Can you work these out from the model? Positions are in its coordinate system, mm. Face numbers are marked on the shaded views. A direction names the side the tool comes from. Give positions to 0.01 mm unless a question says otherwise; leave off trailing zeros. Loops run counter-clockwise (first coordinate to the right, second up) from the corner with the lowest first, then second, coordinate; pieces in that order, holes last. Notation, with made-up numbers: (-35.75, -10.5) -> (-27.75, -10.5) arc R25 cw to (-27.75, 20.5) -> close; hole circle Ø1 at (16.25, 67). An arc over 180 degrees is marked (long way). Return JSON: item names as keys, results as strings. Group by question number.
Q1. Will these pins go through, and if not, where does the flat tip stop? pin 1 (0.6 mm diameter, centred on x = 0.5, y = 4.5, fed in from +Z); pin 2 (6 mm diameter, centred on x = -1.5, y = 2.5, fed in from -Z); pin 3 (1.5 mm diameter, centred on y = -2.5, z = 11, fed in from -X); pin 4 (1.5 mm diameter, centred on y = 4, z = 11, fed in from +X).
Q2. Which directions (+Z, -Z, +X, -X, +Y, -Y) give clear straight access to the entire face, cutting with the end or side of a thin tool? Please do the marked faces 4, 5 and 6.
Q3. Suppose I cut it at B-B, the plane z = 10.25. Please give me the cut outline in (x, y), and give its area (3 significant figures).
Q4. Suppose I cut it at D-D, the plane z = 1. Please give me the cut outline in (x, y).
Q5. I need wall thicknesses on line 1 along Y through (x, z) = (-4.5, 12.75); line 2 along X through (y, z) = (0, 12.5); line 3 along Y through (x, z) = (0, 6.5). Which ranges of each line are inside material? Lowest first, please. Write a range as [from, to].
Q6. Suppose I cut it at C-C, the plane z = 13.25. Count the separate pieces of the cut face and the enclosed holes in it, and give its area (3 significant figures).
Q7. Thinking about a two-plate mould opening in X: for the marked faces 1, 2 and 3, which applies, pulls with the +X half, pulls with the -X half, needs draft (parallel to the pull), parting line crosses it, or undercut?
Q8. Suppose I cut it at A-A, the plane y = 0. Please give me the cut outline in (x, z).
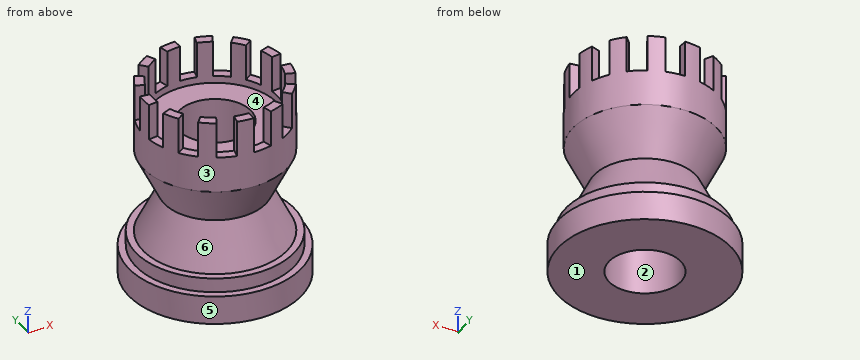
```python
from build123d import *

# Parameters (mm, degrees)
SKETCH_1_R          = 6
EXTRUDE_1_DEPTH     = 2
SKETCH_2_R          = 5.5
EXTRUDE_2_DEPTH     = 1
SKETCH_3_R          = 5
EXTRUDE_3_DEPTH     = 3
EXTRUDE_3_TAPER     = 26
SKETCH_4_R          = 3.536802234
EXTRUDE_4_DEPTH     = 3
EXTRUDE_4_DRAFT     = -26
SKETCH_5_R          = 5
EXTRUDE_5_DEPTH     = 5
SKETCH_6_R          = 4.35308232
CUT_EXTRUDE_1_DEPTH = 3
CUT_EXTRUDE_2_DEPTH = 2.5
SKETCH_8_R          = 2.5
CUT_EXTRUDE_3_DEPTH = 14.892443989


with BuildPart() as part:
    # 스케치1 → 보스-돌출1 (new body)
    with BuildSketch(Plane.XY):
        Circle(SKETCH_1_R)
    extrude(amount=EXTRUDE_1_DEPTH)

    # 스케치2 → 보스-돌출2 (add)
    with BuildSketch(Plane.XY.offset(2)):
        Circle(SKETCH_2_R)
    extrude(amount=EXTRUDE_2_DEPTH)

    # 스케치3 → 보스-돌출3 (add)
    with BuildSketch(Plane.XY.offset(3)):
        Circle(SKETCH_3_R)
    extrude(amount=EXTRUDE_3_DEPTH, taper=EXTRUDE_3_TAPER)


with BuildPart() as extrude_4_tool:
    # 스케치4 → 보스-돌출4 (with draft: the straight prism first)
    with BuildSketch(Plane.XY.offset(6)):
        Circle(SKETCH_4_R)
    extrude(amount=EXTRUDE_4_DEPTH)
    # 보스-돌출4: the draft: its side faces are tilted about the plane it starts from
    extrude_4_sides = [extrude_4_tool.faces().sort_by_distance(p)[0] for p in [
        (-3.536802234, 0, 7.5),
    ]]
    draft(extrude_4_sides, Plane.XY.offset(6), EXTRUDE_4_DRAFT)


with BuildPart() as part_1:
    add(part.part)

    # 보스-돌출4: add extrude_4_tool
    add(extrude_4_tool.part)

    # 스케치5 → 보스-돌출5 (add)
    with BuildSketch(Plane.XY.offset(9)):
        Circle(SKETCH_5_R)
    extrude(amount=EXTRUDE_5_DEPTH)

    # 스케치6 → 컷-돌출1 (cut)
    with BuildSketch(Plane.XY.offset(14)):
        Circle(SKETCH_6_R)
    extrude(amount=-CUT_EXTRUDE_1_DEPTH, mode=Mode.SUBTRACT)

    # 스케치7 → 컷-돌출2 (cut)
    with BuildSketch(Plane.XY.offset(14)):
        with BuildLine():
            Line((0, 4.35308232), (0, 5))
            ThreePointArc((0, 5), (0.642664488, 4.958526228), (1.274667489, 4.834792942))
            Line((1.274667489, 4.834792942), (1.109746502, 4.209250336))
            ThreePointArc((1.109746502, 4.209250336), (0.559514284, 4.316974572), (0, 4.35308232))
        make_face()
        with BuildLine():
            Line((2.022978224, 3.854462971), (2.32361586, 4.427280128))
            ThreePointArc((2.32361586, 4.427280128), (2.873393181, 4.091895847), (3.375502321, 3.688629025))
            Line((3.375502321, 3.688629025), (2.938767895, 3.211381159))
            ThreePointArc((2.938767895, 3.211381159), (2.501623411, 3.562471894), (2.022978224, 3.854462971))
        make_face()
        with BuildLine():
            Line((3.582516517, 2.472832606), (4.114919329, 2.840323734))
            ThreePointArc((4.114919329, 2.840323734), (4.445862124, 2.287861441), (4.70305025, 1.697444651))
            Line((4.70305025, 1.697444651), (4.094552979, 1.47782326))
            ThreePointArc((4.094552979, 1.47782326), (3.870640762, 1.991849838), (3.582516517, 2.472832606))
        make_face()
        with BuildLine():
            Line((4.321343449, 0.524706092), (4.96354437, 0.602683401))
            ThreePointArc((4.96354437, 0.602683401), (4.999837633, -0.04029445), (4.953186046, -0.682603837))
            Line((4.953186046, -0.682603837), (4.312325321, -0.594286139))
            ThreePointArc((4.312325321, -0.594286139), (4.352940961, -0.035081012), (4.321343449, 0.524706092))
        make_face()
        with BuildLine():
            Line((4.070202675, -1.543624265), (4.675081213, -1.773024435))
            ThreePointArc((4.675081213, -1.773024435), (4.408410595, -2.359219368), (4.06860661, -2.906276011))
            Line((4.06860661, -2.906276011), (3.542195901, -2.530251744))
            ThreePointArc((3.542195901, -2.530251744), (3.838034844, -2.053975224), (4.070202675, -1.543624265))
        make_face()
        with BuildLine():
            Line((2.88662752, -3.258328904), (3.315613291, -3.742553741))
            ThreePointArc((3.315613291, -3.742553741), (2.807069816, -4.137675561), (2.251958432, -4.464155376))
            Line((2.251958432, -4.464155376), (1.960592088, -3.886567168))
            ThreePointArc((1.960592088, -3.886567168), (2.443881198, -3.602328466), (2.88662752, -3.258328904))
        make_face()
        with BuildLine():
            Line((1.041760787, -4.22658966), (1.196578321, -4.854709087))
            ThreePointArc((1.196578321, -4.854709087), (0.562663172, -4.968240147), (-0.080586283, -4.999350543))
            Line((-0.080586283, -4.999350543), (-0.070159745, -4.352516892))
            ThreePointArc((-0.070159745, -4.352516892), (0.489863821, -4.325431669), (1.041760787, -4.22658966))
        make_face()
        with BuildLine():
            Line((-1.041760787, -4.22658966), (-1.196578321, -4.854709087))
            ThreePointArc((-1.196578321, -4.854709087), (-1.810642825, -4.660640789), (-2.394669653, -4.389254749))
            Line((-2.394669653, -4.389254749), (-2.084838826, -3.82135745))
            ThreePointArc((-2.084838826, -3.82135745), (-1.576375454, -4.057630604), (-1.041760787, -4.22658966))
        make_face()
        with BuildLine():
            Line((-2.88662752, -3.258328904), (-3.315613291, -3.742553741))
            ThreePointArc((-3.315613291, -3.742553741), (-3.76915237, -3.285344793), (-4.160163063, -2.773633589))
            Line((-4.160163063, -2.773633589), (-3.621906456, -2.414771068))
            ThreePointArc((-3.621906456, -2.414771068), (-3.281486109, -2.860275267), (-2.88662752, -3.258328904))
        make_face()
        with BuildLine():
            Line((-4.070202675, -1.543624265), (-4.675081213, -1.773024435))
            ThreePointArc((-4.675081213, -1.773024435), (-4.864194531, -1.157415898), (-4.972613252, -0.522606399))
            Line((-4.972613252, -0.522606399), (-4.329238966, -0.454989735))
            ThreePointArc((-4.329238966, -0.454989735), (-4.234847844, -1.007665336), (-4.070202675, -1.543624265))
        make_face()
        with BuildLine():
            Line((-4.321343449, 0.524706092), (-4.96354437, 0.602683401))
            ThreePointArc((-4.96354437, 0.602683401), (-4.844908345, 1.235663031), (-4.645897671, 1.848143618))
            Line((-4.645897671, 1.848143618), (-4.044795002, 1.609024262))
            ThreePointArc((-4.044795002, 1.609024262), (-4.218056972, 1.075788579), (-4.321343449, 0.524706092))
        make_face()
        with BuildLine():
            Line((-3.582516517, 2.472832606), (-4.114919329, 2.840323734))
            ThreePointArc((-4.114919329, 2.840323734), (-3.715712045, 3.345666451), (-3.254862922, 3.795506206))
            Line((-3.254862922, 3.795506206), (-2.833737248, 3.304430192))
            ThreePointArc((-2.833737248, 3.304430192), (-3.234960082, 2.912792296), (-3.582516517, 2.472832606))
        make_face()
        with BuildLine():
            Line((-2.022978224, 3.854462971), (-2.32361586, 4.427280128))
            ThreePointArc((-2.32361586, 4.427280128), (-1.735290894, 4.689218007), (-1.118178304, 4.873364062))
            Line((-1.118178304, 4.873364062), (-0.973504441, 4.242830988))
            ThreePointArc((-0.973504441, 4.242830988), (-1.510772822, 4.0825104), (-2.022978224, 3.854462971))
        make_face()
    extrude(amount=-CUT_EXTRUDE_2_DEPTH, mode=Mode.SUBTRACT)

    # 스케치8 → 컷-돌출3 (cut, through all)
    with BuildSketch(Plane.XY.offset(11)):
        Circle(SKETCH_8_R)
    extrude(amount=-CUT_EXTRUDE_3_DEPTH, mode=Mode.SUBTRACT)


solid = part_1.part
```
Ans:
{
 "1": {"pin 1": "stops at z = 11.5", "pin 2": "stops at z = 0", "pin 3": "stops at x = -4.68", "pin 4": "stops at x = 3.8"},
 "2": {"face 4": "+Z", "face 5": "+Z, -Z", "face 6": "none"},
 "3": {"outline": "circle Ø10 at (0, 0); hole circle Ø5 at (0, 0)", "area": "58.9 mm^2"},
 "4": {"outline": "circle Ø12 at (0, 0); hole circle Ø5 at (0, 0)"},
 "5": {"line 1": "y = [-2.18, -1.71], [-0.47, 0.55], [1.79, 2.18]", "line 2": "x = [-5, -4.35]", "line 3": "y = [-3.78, -2.5], [2.5, 3.78]"},
 "6": {"separate pieces": "13", "enclosed holes": "0", "area": "8.87 mm^2"},
 "7": {"face 1": "needs draft", "face 2": "undercut", "face 3": "parting line crosses it"},
 "8": {"outline": "(-6, 0) -> (-2.5, 0) -> (-2.5, 11) -> (-4.35, 11) -> (-4.35, 14) -> (-5, 14) -> (-5, 9) -> (-3.54, 6) -> (-5, 3) -> (-5.5, 3) -> (-5.5, 2) -> (-6, 2) -> close; (2.5, 0) -> (6, 0) -> (6, 2) -> (5.5, 2) -> (5.5, 3) -> (5, 3) -> (3.54, 6) -> (5, 9) -> (5, 11.5) -> (4.35, 11.5) -> (4.35, 11) -> (2.5, 11) -> close"}
}
